For this review, take the finished solid that the model builds, in its own axes (mm). A direction names the side the tool comes from. Round coordinates to 2 decimals unless told otherwise and drop trailing zeros. Loops run counter-clockwise (first coordinate to the right, second up) from the corner with the lowest first, then second, coordinate; pieces in that order, holes last. Notation, with made-up numbers: M 70.5,24 L 113.5,24 A16 cw 113.5,48 Z; hole C -39.75,14.25 d1. An arc over 180 degrees is marked long. Write item = value, one per line. Start each with the question number.
```python
from build123d import *

# Parameters (mm, degrees)
SKETCH_1_R      = 3.4
EXTRUDE_1_DEPTH = 100


with BuildPart() as part:
    # 草图1 → 凸台-拉伸1 (new body)
    with BuildSketch(Plane.XY):
        with BuildLine():
            Line((-23.338979522, 16.722515545), (-23.338979522, 4.394054978))
            Line((-23.338979522, 4.394054978), (-22.538979522, 4.394054978))
            ThreePointArc((-22.538979522, 4.394054978), (-22.397558165, 4.335476334), (-22.338979522, 4.194054978))
            Line((-22.338979522, 4.194054978), (-22.338979522, 3.394054978))
            Line((-22.338979522, 3.394054978), (-19.138979522, 3.394054978))
            ThreePointArc((-19.138979522, 3.394054978), (-18.926847487, 3.481922943), (-18.838979522, 3.694054978))
            Line((-18.838979522, 3.694054978), (-18.838979522, 5.594054978))
            ThreePointArc((-18.838979522, 5.594054978), (-18.926847487, 5.806187012), (-19.138979522, 5.894054978))
            Line((-19.138979522, 5.894054978), (-20.338979522, 5.894054978))
            ThreePointArc((-20.338979522, 5.894054978), (-21.046086303, 6.186948197), (-21.338979522, 6.894054978))
            Line((-21.338979522, 6.894054978), (-21.338979522, 8.544054978))
            ThreePointArc((-21.338979522, 8.544054978), (-21.046086303, 9.251161759), (-20.338979522, 9.544054978))
            Line((-20.338979522, 9.544054978), (-15.356746475, 9.544054978))
            Line((-15.356746475, 9.544054978), (-11.038979522, 5.226288025))
            Line((-11.038979522, 5.226288025), (-11.038979522, -6.638178069))
            Line((-11.038979522, -6.638178069), (-15.356746475, -10.955945022))
            Line((-15.356746475, -10.955945022), (-20.338979522, -10.955945022))
            ThreePointArc((-20.338979522, -10.955945022), (-21.046086303, -10.663051803), (-21.338979522, -9.955945022))
            Line((-21.338979522, -9.955945022), (-21.338979522, -8.305945022))
            ThreePointArc((-21.338979522, -8.305945022), (-21.046086303, -7.598838241), (-20.338979522, -7.305945022))
            Line((-20.338979522, -7.305945022), (-19.138979522, -7.305945022))
            ThreePointArc((-19.138979522, -7.305945022), (-18.926847487, -7.218077057), (-18.838979522, -7.005945022))
            Line((-18.838979522, -7.005945022), (-18.838979522, -5.105945022))
            ThreePointArc((-18.838979522, -5.105945022), (-18.926847487, -4.893812988), (-19.138979522, -4.805945022))
            Line((-19.138979522, -4.805945022), (-22.338979522, -4.805945022))
            Line((-22.338979522, -4.805945022), (-22.338979522, -5.605945022))
            ThreePointArc((-22.338979522, -5.605945022), (-22.397558165, -5.747366379), (-22.538979522, -5.805945022))
            Line((-22.538979522, -5.805945022), (-23.338979522, -5.805945022))
            Line((-23.338979522, -5.805945022), (-23.338979522, -17.205945022))
            ThreePointArc((-23.338979522, -17.205945022), (-22.313853256, -19.680818756), (-19.838979522, -20.705945022))
            Line((-19.838979522, -20.705945022), (-8.438979522, -20.705945022))
            Line((-8.438979522, -20.705945022), (-8.438979522, -19.905945022))
            ThreePointArc((-8.438979522, -19.905945022), (-8.380400878, -19.764523666), (-8.238979522, -19.705945022))
            Line((-8.238979522, -19.705945022), (-7.438979522, -19.705945022))
            Line((-7.438979522, -19.705945022), (-7.438979522, -16.505945022))
            ThreePointArc((-7.438979522, -16.505945022), (-7.526847487, -16.293812988), (-7.738979522, -16.205945022))
            Line((-7.738979522, -16.205945022), (-9.638979522, -16.205945022))
            ThreePointArc((-9.638979522, -16.205945022), (-9.851111556, -16.293812988), (-9.938979522, -16.505945022))
            Line((-9.938979522, -16.505945022), (-9.938979522, -17.705945022))
            ThreePointArc((-9.938979522, -17.705945022), (-10.231872741, -18.413051803), (-10.938979522, -18.705945022))
            Line((-10.938979522, -18.705945022), (-12.588979522, -18.705945022))
            ThreePointArc((-12.588979522, -18.705945022), (-13.296086303, -18.413051803), (-13.588979522, -17.705945022))
            Line((-13.588979522, -17.705945022), (-13.588979522, -12.723711975))
            Line((-13.588979522, -12.723711975), (-9.271212569, -8.405945022))
            Line((-9.271212569, -8.405945022), (2.593253525, -8.405945022))
            Line((2.593253525, -8.405945022), (6.911020478, -12.723711975))
            Line((6.911020478, -12.723711975), (6.911020478, -17.705945022))
            ThreePointArc((6.911020478, -17.705945022), (6.618127259, -18.413051803), (5.911020478, -18.705945022))
            Line((5.911020478, -18.705945022), (4.261020478, -18.705945022))
            ThreePointArc((4.261020478, -18.705945022), (3.553913697, -18.413051803), (3.261020478, -17.705945022))
            Line((3.261020478, -17.705945022), (3.261020478, -16.505945022))
            ThreePointArc((3.261020478, -16.505945022), (3.173152513, -16.293812988), (2.961020478, -16.205945022))
            Line((2.961020478, -16.205945022), (1.061020478, -16.205945022))
            ThreePointArc((1.061020478, -16.205945022), (0.848888444, -16.293812988), (0.761020478, -16.505945022))
            Line((0.761020478, -16.505945022), (0.761020478, -19.705945022))
            Line((0.761020478, -19.705945022), (1.561020478, -19.705945022))
            ThreePointArc((1.561020478, -19.705945022), (1.702441835, -19.764523666), (1.761020478, -19.905945022))
            Line((1.761020478, -19.905945022), (1.761020478, -20.705945022))
            Line((1.761020478, -20.705945022), (14.089481045, -20.705945022))
            ThreePointArc((14.089481045, -20.705945022), (15.826995028, -20.003455845), (16.588041197, -18.290781149))
            ThreePointArc((16.588041197, -18.290781149), (4.945291726, 7.578326225), (-20.923815648, 19.221075696))
            ThreePointArc((-20.923815648, 19.221075696), (-22.636490345, 18.460029528), (-23.338979522, 16.722515545))
        make_face()
        with Locations((-3.338979522, -0.705945022)):
            Circle(SKETCH_1_R, mode=Mode.SUBTRACT)
        with BuildLine():
            Line((-15.088979522, -13.455945022), (-15.088979522, -18.209945022))
            ThreePointArc((-15.088979522, -18.209945022), (-15.381872741, -18.917051803), (-16.088979522, -19.209945022))
            Line((-16.088979522, -19.209945022), (-19.342979522, -19.209945022))
            ThreePointArc((-19.342979522, -19.209945022), (-21.110746475, -18.477711975), (-21.842979522, -16.709945022))
            Line((-21.842979522, -16.709945022), (-21.842979522, -13.455945022))
            ThreePointArc((-21.842979522, -13.455945022), (-21.550086303, -12.748838241), (-20.842979522, -12.455945022))
            Line((-20.842979522, -12.455945022), (-16.088979522, -12.455945022))
            ThreePointArc((-16.088979522, -12.455945022), (-15.381872741, -12.748838241), (-15.088979522, -13.455945022))
        make_face(mode=Mode.SUBTRACT)
        with BuildLine():
            Line((-15.776737791, 11.544054978), (-21.038979522, 11.544054978))
            ThreePointArc((-21.038979522, 11.544054978), (-21.251111556, 11.631922943), (-21.338979522, 11.844054978))
            Line((-21.338979522, 11.844054978), (-21.338979522, 16.923830422))
            ThreePointArc((-21.338979522, 16.923830422), (-21.244538861, 17.142337534), (-21.020677134, 17.223271606))
            ThreePointArc((-21.020677134, 17.223271606), (3.531078163, 6.164112663), (14.590237107, -18.387642635))
            ThreePointArc((14.590237107, -18.387642635), (14.509303035, -18.611504361), (14.290795923, -18.705945022))
            Line((14.290795923, -18.705945022), (9.211020478, -18.705945022))
            ThreePointArc((9.211020478, -18.705945022), (8.998888444, -18.618077057), (8.911020478, -18.405945022))
            Line((8.911020478, -18.405945022), (8.911020478, -13.143703291))
            ThreePointArc((8.911020478, -13.143703291), (8.777145631, -11.512883109), (8.379105585, -9.925728086))
            ThreePointArc((8.379105585, -9.925728086), (0.349097648, 2.982132147), (-12.558762586, 11.012140084))
            ThreePointArc((-12.558762586, 11.012140084), (-14.145917608, 11.410180131), (-15.776737791, 11.544054978))
        make_face(mode=Mode.SUBTRACT)
    extrude(amount=EXTRUDE_1_DEPTH)


solid = part.part
```
(1) For pin 1 Ø1.8 at (x, z) = (-12, 48.5) entering from +Y; pin 2 Ø1 at (y, z) = (-17, 36) entering from +X; pin 3 Ø9.5 at (y, z) = (-0.5, 30.5) entering from -X, all flat-tipped, find the tip position at first contact; note any pin that passes through.
(2) Wall thickness on L1, parallel to X at y = 7.5, z = 11.5; L2, parallel to X at y = 7, z = 80; L3, parallel to Y at x = -15, z = 10: over which ranges is each line inside the solid? List them lowest first.
(3) Add section D-D on z = 41. Count the separate pieces of the cut face and the enclosed holes in it, and give its area (3 significant figures).
(4) Tool access review of faces 1 (the flat face through (12, -18.706, 49)), 2 (the cylindrical face through (-22.341, -19.653, 49.3)), 3 (the flat face through (-21, -4.806, 49)), 4 (the flat face through (-7.439, -18, 49)), 5 (the flat face through (-23.339, 11, 49)): name each direction out of +Z, -Z, +X, -X, +Y, -Y from which nothing blocks a thin tool from reaching the whole face with its end or side.
(5) Add section B-B on x = 12.5. Write out the cut boundary in (y, z), and give its area (3 significant figures).
(6) Add section C-C on x = -1.5. Write out the cut boundary in (y, z).
(7) Add section A-A on y = -15. Write out the cut boundary in (x, z).
(8) Draft analysis for pull direction X (two halves, no side actions). For faces 6 (the flat face through (-21.843, -15, 49)), 7 (the cylindrical face through (-22.618, 18.479, 49.3)), 8 (the flat face through (8, -20.706, 49)), state which applies: +X half, -X half, draft (parallel to the pull), parting line (faces both ways), or undercut.
Answer sheet:
q1.pin_1 = 17.91
q1.pin_2 = 16.53
q1.pin_3 = -22.35
q2.L1 = -23.34 to -21.34, -13.31 to -5.26, 2.13 to 5.02
q2.L2 = -23.34 to -21.34, -12.81 to -4.51, 2.67 to 5.51
q2.L3 = -20.71 to -10.6, 9.19 to 11.51, 16.37 to 18.42
q3.separate_pieces = 1
q3.enclosed_holes = 3
q3.area = 531 mm²
q4.face_1 = +Z, -Z
q4.face_2 = +Z, -Z, -X, -Y
q4.face_3 = +Z, -Z, -X
q4.face_4 = +Z, -Z, -Y
q4.face_5 = +Z, -Z, -X, +Y, -Y
q5.outline = M -20.71,0 L -18.71,0 L -18.71,100 L -20.71,100 Z; M -8.07,0 L -2.94,0 L -2.94,100 L -8.07,100 Z
q5.area = 713 mm²
q6.outline = M -8.41,0 L -3.57,0 L -3.57,100 L -8.41,100 Z; M 2.15,0 L 4.7,0 L 4.7,100 L 2.15,100 Z; M 10.39,0 L 12.81,0 L 12.81,100 L 10.39,100 Z
q7.outline = M -23.34,0 L -21.84,0 L -21.84,100 L -23.34,100 Z; M -15.09,0 L -13.59,0 L -13.59,100 L -15.09,100 Z; M 6.91,0 L 8.91,0 L 8.91,100 L 6.91,100 Z; M 14.23,0 L 16.25,0 L 16.25,100 L 14.23,100 Z
q8.face_6 = undercut
q8.face_7 = -X half
q8.face_8 = draft
